The listing builds one solid part. Answer for the finished solid, in the listing's coordinates (mm). A direction names the side the tool comes from. Coordinates: 2 decimals unless noted, no trailing zeros. Write each loop counter-clockwise with the first axis right and the second up, starting at its lowest first coordinate (ties: lowest second). Pieces come first, ordered by that corner, then holes. Notation, with made-up numbers: M 18.25,68 L 56.25,68 A20 ccw 56.25,100 Z; hole C -9,43 d2. An arc over 180 degrees is marked long. Answer as CSV lines item,"result".
Autodesk Inventor part; units mm, degrees
ref_plane "YZ Plane" through (0, 0, 0) normal (1, 0, 0) x (0, 1, 0)
ref_plane "XZ Plane" through (0, 0, 0) normal (0, 1, 0) x (-1, 0, 0)
ref_plane "XY Plane" through (0, 0, 0) normal (0, 0, 1) x (1, 0, 0)
ref_plane "Work Plane1" through (0, 0, 0) normal (0, 0, 1) x (1, 0, 0)
sketch "Sketch1" plane through (0, 0, 0) normal (0, 0, 1) x (1, 0, 0)
  circle A0 centre (-10, -25) radius 1.45
  circle A1 centre (-10, 25) radius 1.45
  circle A2 centre (10, 25) radius 1.45
  circle A3 centre (10, -25) radius 1.45
  circle A4 centre (-25, 25) radius 2.325
  circle A5 centre (25, -25) radius 2.325
  circle A6 centre (-25, -25) radius 2.325
  circle A7 centre (25, 25) radius 2.325
  line L0 (28, 30) -> (30, 28)
  line L1 (28, 30) -> (-28, 30)
  line L2 (-30, 28) -> (-28, 30)
  line L3 (-30, 28) -> (-30, -28)
  line L4 (-28, -30) -> (-30, -28)
  line L5 (-28, -30) -> (28, -30)
  line L6 (30, -28) -> (28, -30)
  line L7 (30, -28) -> (30, 28)
  circle A8 centre (-17.5, -17.5) radius 1.95
  circle A9 centre (17.5, 17.5) radius 1.95
  circle A10 centre (17.5, -17.5) radius 1.95
  circle A11 centre (-17.5, 17.5) radius 1.95
  circle A12 centre (0, 0) radius 7.5
  circle A13 centre (-25.33, -75.26) radius 6.15
  circle A14 centre (25, -10) radius 1.45
  circle A15 centre (-25, -10) radius 1.45
  circle A16 centre (-25, 10) radius 1.45
  circle A17 centre (25, 10) radius 1.45
  line L8 (-30, -28) -> (-30, -30)
  line L9 (-30, -30) -> (-28, -30)
  point P0 (0, 0)
extrude "Extrusion1" add sketch "Sketch1" along normal blind 8 contours L0 L7 L6 L5 L4 L3 L2 L1 | L4 L9 L8
sketch "Sketch2" plane through (0, 0, 8) normal (0, 0, 1) x (1, 0, 0)
  circle A0 centre (0, 0) radius 7.5
  circle A1 centre (25, 10) radius 1.45
  circle A2 centre (-25, 10) radius 1.45
  circle A3 centre (-25, -10) radius 1.45
  circle A4 centre (25, -10) radius 1.45
  circle A5 centre (10, -25) radius 1.45
  circle A6 centre (10, 25) radius 1.45
  circle A7 centre (-10, 25) radius 1.45
  circle A8 centre (-10, -25) radius 1.45
  line L0 (-30, -30) -> (28, -30)
  line L1 (28, -30) -> (30, -28)
  line L2 (30, -28) -> (30, 28)
  line L3 (30, 28) -> (28, 30)
  line L4 (28, 30) -> (-28, 30)
  line L5 (30, -28) -> (30, 28)
  line L6 (30, 28) -> (30, -28)
  line L7 (-28, 30) -> (-30, 28)
  line L8 (-30, 28) -> (-30, -30)
  line L9 (-30, -30) -> (-18, -30)
  line L10 (-18, -30) -> (-18, -80)
  line L11 (-18, -80) -> (-30, -80)
  line L12 (-30, -80) -> (-30, -30)
  line L13 (-30, -30) -> (-30, -28)
  line L14 (-30, -28) -> (-28, -30)
  line L15 (-28, -30) -> (-30, -30)
  circle A9 centre (-17.5, 17.5) radius 1.95
  circle A10 centre (-25, 25) radius 2.325
  circle A11 centre (25, 25) radius 2.325
  circle A12 centre (17.5, 17.5) radius 1.95
  circle A13 centre (17.5, -17.5) radius 1.95
  circle A14 centre (25, -25) radius 2.325
  circle A15 centre (-25, -25) radius 2.325
  line L16 (-30, -80) -> (30, -80)
  line L17 (30, -80) -> (30, -92)
  line L18 (30, -92) -> (-30, -92)
  line L19 (-30, -92) -> (-30, -80)
  point P0 (0, 0)
  point P1 (-24.2387, -104)
  dimension "d59" = 12
  dimension "d77" = 12
extrude "Extrusion2" add sketch "Sketch2" along normal blind 7 contours A0 | A1 | A2 | A3 | A4 | A5 | A6 | A7 | A8 | L8 L14 L0 | L0 L10 L11 L12 | L14 L8 L7 L4 L3 L2 L1 L0 | L11 L16 L17 L18 L19 | A9 | A10 | A11 | A12 | A13 | A14 | A15
fillet "Fillet1" radius 4 5 edges at (-18, -30, 11.5) (-30, -92, 11.5) (30, -92, 11.5) (30, -80, 11.5) (-18, -80, 11.5)
sketch "Sketch6" plane through (0, 0, 15) normal (0, 0, 1) x (1, 0, 0)
  line L0 (30, -28) -> (30, 28)
  line L1 (30, 28) -> (28, 30)
  line L2 (28, 30) -> (-28, 30)
  circle A0 centre (-1.1442, -37.6316) radius 2.45
  circle A1 centre (-1.1442, -37.6316) radius 1.45 construction
  line L3 (-14, -30) -> (28, -30)
  line L4 (-28, 30) -> (-30, 28)
  line L5 (-18, -76) -> (-18, -34)
  arc A2 (-14, -30) -> (-18, -34) centre (-14, -34) ccw
  line L6 (-26, -92) -> (26, -92)
  line L7 (30, -88) -> (30, -84)
  line L8 (26, -80) -> (-14, -80)
  line L9 (28, -30) -> (30, -28)
  arc A3 (30, -84) -> (26, -80) centre (26, -84) ccw
  arc A4 (-18, -76) -> (-14, -80) centre (-14, -76) ccw
  arc A5 (-30, -88) -> (-26, -92) centre (-26, -88) ccw
  arc A6 (26, -92) -> (30, -88) centre (26, -88) ccw
  line L10 (-30, 28) -> (-30, -88)
  point P0 (0, 0)
  dimension "d27" = 4.9
extrude "Extrusion6" cut sketch "Sketch6" against normal blind 4 contours A0
ref_plane "Work Plane2" through (-6, -91, 19) normal (1, 0, 0) x (0, 0, -1)
sketch "Sketch7" plane through (0, 0, 15) normal (0, 0, 1) x (1, 0, 0)
  circle A0 centre (10, -25) radius 1.45
  circle A1 centre (-10, -25) radius 1.45
  circle A2 centre (-25, -10) radius 1.45
  circle A3 centre (-25, 10) radius 1.45
  circle A4 centre (-10, 25) radius 1.45
  circle A5 centre (10, 25) radius 1.45
  circle A6 centre (25, 10) radius 1.45
  circle A7 centre (25, -10) radius 1.45
  circle A8 centre (-25, 25) radius 2.325
  circle A9 centre (25, 25) radius 2.325
  circle A10 centre (25, -25) radius 2.325
  circle A11 centre (-25, -25) radius 2.325
  point P0 (0, 0)
hole "Hole1" at (-25, -10, 15) at (-25, 10, 15) at (-10, 25, 15) at (10, 25, 15) at (25, 10, 15) at (25, -10, 15) at (10, -25, 15) at (-10, -25, 15) at (-25, 25, 15) at (-25, -25, 15) at (25, -25, 15) at (25, 25, 15) direction (0, 0, -1) diameter 3.2 end through all counterbore diameter 8 counterbore depth 10
sketch "Sketch8" plane through (0, 0, 15) normal (0, 0, 1) x (1, 0, 0)
  circle A0 centre (0, 0) radius 16
  dimension "d41" = 32
extrude "Extrusion7" cut sketch "Sketch8" against normal through all
chamfer "Chamfer3" distance 5 angle 75 1 edges at (-22, -30, 8) measured on face at (14, -30, 7.6667)
properties part number "cellSTORM_UC2_Sample_arm"
Q1. Find section B-B (y = -10). Give the vertices of the cut face in (x, z), and give its area (3 significant figures).
Output:
outline,"M -30,0 L -26.6,0 L -26.6,5 L -29,5 L -29,15 L -30,15 Z; M -23.4,0 L -12.49,0 L -12.49,15 L -21,15 L -21,5 L -23.4,5 Z; M 12.49,0 L 23.4,0 L 23.4,5 L 21,5 L 21,15 L 12.49,15 Z; M 26.6,0 L 30,0 L 30,15 L 29,15 L 29,5 L 26.6,5 Z"
area,"333 mm2"
Q2. The mould has two halves that part along X. Classify faces 4 (the cylindrical face through (-16.859, -78.797, 11.549)), 5 (the flat face through (-14, 14, 0)), 6 (the cylindrical face through (15.953, 18.687, 3.944)): pulls with the +X half, pulls with the -X half, needs draft (parallel to the pull), parting line crosses it, or undercut.
Output:
face 4,"pulls with the +X half"
face 5,"needs draft"
face 6,"undercut"
Q3. Flat-ended cylindrical pins translate along their axes: pin 1 Ø2.5 at (x, y) = (-10, -25) entering from +Z; pin 2 Ø1.2 at (x, y) = (18, 18) entering from -Z; pin 3 Ø5 at (x, z) = (21, 2.5) entering from -Y; pin 4 Ø4 at (x, y) = (-9.5, 26) entering from +Z. Find the tip coordinate at first contact, or state that the pin passes through.
Output:
pin 1,"through"
pin 2,"z = 8"
pin 3,"y = -30"
pin 4,"z = 5"
Q4. For faces 1 (the flat face through (17, -17, 8)), 2 (the flat face through (10, -27, 5)), 3 (the cylindrical face through (-8.44, -24.65, 2.46)), determine the directions among +Z, -Z, +X, -X, +Y, -Y from which every point of the face is accessible in a straight line to the end or side of a thin tool.
Output:
face 1,"-Z"
face 2,"+Z"
face 3,"+Z, -Z"
Q5. Find section C-C (z = 13.5). Count the separate pieces of the cut face and the enclosed holes in it, and give its area (3 significant figures).
Output:
separate pieces,"1"
enclosed holes,"13"
area,"3,500 mm2"
Q6. Find section D-D (x = 17.5). Give the vertices of the cut face in (y, z), and give its area (3 significant figures).
Output:
outline,"M -92,8 L -80,8 L -80,15 L -92,15 Z; M -30,0 L -19.45,0 L -19.45,8 L -15.55,8 L -15.55,0 L 15.55,0 L 15.55,8 L 19.45,8 L 19.45,0 L 30,0 L 30,15 L -30,15 Z"
area,"922 mm2"
Q7. Find section A-A (x = 0). Give the vertices of the cut face in (y, z).
Output:
outline,"M -92,8 L -80,8 L -80,15 L -92,15 Z; M -30,0 L -16,0 L -16,15 L -30,15 Z; M 16,0 L 30,0 L 30,15 L 16,15 Z"
Q8. Straight lines are drawn through the part: line 1 (Y direction, x = -25, z = 2.9) (3 decimals); line 2 (Y direction, x = -25, z = 9); line 3 (X direction, y = 25, z = 10.5). For each, find the intervals that lie inside material, in ascending order.
Output:
line 1,"-30 to -27.325, -22.675 to -11.6, -8.4 to 8.4, 11.6 to 22.675, 27.325 to 30"
line 2,"-92 to -29, -21 to -14, -6 to 6, 14 to 21, 29 to 30"
line 3,"-30 to -29, -21 to -14, -6 to 6, 14 to 21, 29 to 30"
